from build123d import *

# Parameters (mm, degrees)
SKETCH1_R           = 20
SKETCH1_R_2         = 12
BOSS_EXTRUDE1_DEPTH = 73
BOSS_EXTRUDE2_REACH = 57
SKETCH2_W           = 36
SKETCH2_H           = 40
SKETCH2_R           = 11
SKETCH4_W           = 48.323472828
SKETCH4_H           = 8
CUT_EXTRUDE1_DEPTH  = 8
SKETCH5_W           = 42.586033238
SKETCH5_H           = 8
CUT_EXTRUDE2_DEPTH  = 8


with BuildPart() as part:
    # Sketch1 → Boss-Extrude1 (new body)
    with BuildSketch(Plane.XY):
        Circle(SKETCH1_R)
        Circle(SKETCH1_R_2, mode=Mode.SUBTRACT)
    extrude(amount=-BOSS_EXTRUDE1_DEPTH)

    # Sketch2 → Boss-Extrude2 (add, up to next)
    with BuildSketch(Plane(origin=(35, 0, 0), x_dir=(0, 0, -1), z_dir=(1, 0, 0)), mode=Mode.PRIVATE) as boss_extrude2_sk1:
        with Locations((30, 0)):
            Rectangle(SKETCH2_W, SKETCH2_H)
        with Locations((30, -2)):
            Circle(SKETCH2_R, mode=Mode.SUBTRACT)
    boss_extrude2_tool1 = extrude(boss_extrude2_sk1.sketch, amount=-BOSS_EXTRUDE2_REACH, mode=Mode.PRIVATE) - part.part
    add(boss_extrude2_tool1.solids().sort_by_distance((35, -19.461855, -30))[0])

    # Sketch4 → Cut-Extrude1 (cut)
    with BuildSketch(Plane.XY):
        with Locations((-1.709156929, 0)):
            Rectangle(SKETCH4_W, SKETCH4_H)
    extrude(amount=-CUT_EXTRUDE1_DEPTH, mode=Mode.SUBTRACT)

    # Sketch5 → Cut-Extrude2 (cut)
    with BuildSketch(Plane(origin=(0, 0, -73), x_dir=(-1, 0, 0), z_dir=(0, 0, -1))):
        Rectangle(SKETCH5_W, SKETCH5_H)
    extrude(amount=-CUT_EXTRUDE2_DEPTH, mode=Mode.SUBTRACT)


solid = part.part
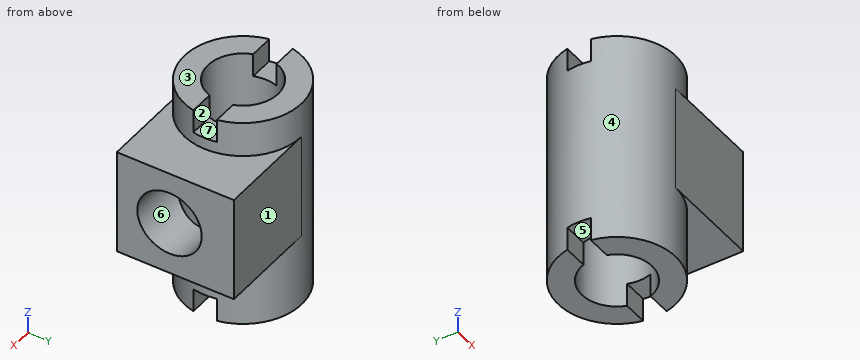
The model under review builds one solid part; all positions refer to its coordinate system, in mm. Face numbers are marked on the shaded views. A direction names the side the tool comes from. Coordinates: 2 decimals unless noted, no trailing zeros. Loops run counter-clockwise (first coordinate to the right, second up) from the corner with the lowest first, then second, coordinate; pieces in that order, holes last.
(1) Tool access review of the marked faces 4, 5, 6 and 7: name each direction out of +Z, -Z, +X, -X, +Y, -Y from which nothing blocks a thin tool from reaching the whole face with its end or side.
Determined:
face 4: none
face 5: -Z, +X, -X
face 6: +X
face 7: +Z, +X, -X
(2) Consider section B-B, the plane y = 5. Give the boundary of the cut face in (x, z), plus the area to 3 significant figures.
Determined:
outline: (-19.36, -73) - (-10.91, -73) - (-10.91, 0) - (-19.36, 0) - close; (10.91, -73) - (19.36, -73) - (19.36, -48) - (35, -48) - (35, -38.49) - (19.36, -38.49) - (19.36, -21.51) - (35, -21.51) - (35, -12) - (19.36, -12) - (19.36, 0) - (10.91, 0) - close
area: 1,530 mm2
(3) Consider section D-D, the plane y = 16. Give the boundary of the cut face in (x, z), plus the area to 3 significant figures.
Determined:
outline: (-12, -73) - (12, -73) - (12, -48) - (35, -48) - (35, -12) - (12, -12) - (12, 0) - (-12, 0) - close
area: 2,580 mm2
(4) Draft analysis for pull direction Y (two halves, no side actions). For the marked faces 1, 2 and 3, state which applies: +Y half, -Y half, draft (parallel to the pull), parting line (faces both ways), or undercut.
Determined:
face 1: +Y half
face 2: undercut
face 3: draft
(5) Wall thickness on L1, parallel to Y at x = 24, z = -30; L2, parallel to Y at x = 0, z = -19; L3, parallel to Z at x = 21, y = -2: over which ranges is each line inside the solid? List them lowest first.
Determined:
L1: y = -20 to -13, 9 to 20
L2: y = -20 to -12, 12 to 20
L3: z = -48 to -41, -19 to -12
(6) Consider section C-C, the plane z = -27. Give the boundary of the cut face in (x, y), plus the area to 3 significant figures.
Determined:
outline: (0, -20) - (35, -20) - (35, -12.58) - (15.55, -12.58) arc R20 ccw to (18.06, 8.58) - (35, 8.58) - (35, 20) - (0, 20) arc R20 ccw to start; hole circle Ø24 at (0, 0)
area: 1,240 mm2
(7) Insertion check: P1, Ø4, axis at x = -11.5, z = -49.5, coming from the -Y side; P2, Ø6.5, axis at x = 17, y = 0.5, coming from the +Z side; P3, Ø8, axis at y = -8, z = -35, coming from the -X side; P4, Ø14.5, axis at x = 0, y = 0, coming from the +Z side. Each pin has a flat end and moves straight along its axis. Give the tip position at first contact, or say it passes through.
Determined:
P1: stops at y = -17.6
P2: stops at z = -8
P3: stops at x = -19.6
P4: passes through
(8) Consider section A-A, the plane x = 24.5. Give the boundary of the cut face in (y, z), plus the area to 3 significant figures.
Determined:
outline: (-20, -48) - (20, -48) - (20, -12) - (-20, -12) - close; hole circle Ø22 at (-2, -30)
area: 1,060 mm2
